Input: part model. Units: mm. Frame: model coordinates. Face numbers are marked on the shaded views. Coordinates: 2 decimals unless noted, no trailing zeros. Write each loop counter-clockwise with the first axis right and the second up, starting at its lowest first coordinate (ties: lowest second). Pieces come first, ordered by that corner, then holes. Notation, with made-up numbers: (-20.5, 31) - (19.5, 31) arc R20 ccw to (19.5, 46) - close; hole circle Ø6 at (41.5, -3). An arc over 180 degrees is marked (long way). One line per question, with ' | ' between items. Start each with the question number.
1) Draft query along Y for the marked faces 1 and 2. Return one class per face: released by +Y, released by -Y, zero draft, split by the parting line, or undercut.
2) First-contact query: P1, Ø1, axis at x = -9, z = 103, coming from the +Y side; P2, Ø5, axis at y = 99, z = 64, coming from the -X side; P3, Ø2.5, axis at x = -9, z = 40.5, coming from the -Y side. Flat tips, straight axial feed; report the tip coordinate or a pass-through.
3) Section query B-B on y = 100. Return loops of the section in (x, z).
4) Line query: line 1 (Y direction, x = -3.9, z = 127.75); line 2 (Z direction, x = -2, y = 79.5); line 3 (X direction, y = 83.5, z = 32.5). Output: solid intervals per line, ascending.
```python
from build123d import *
from OCP.BRepFilletAPI import BRepFilletAPI_MakeChamfer

# Parameters (mm, degrees)
SKETCH1_W           = 95
SKETCH1_H           = 145
BOSS_EXTRUDE1_DEPTH = 10
SKETCH2_W           = 3.3
SKETCH2_H           = 4.8
BOSS_EXTRUDE2_DEPTH = 95
SKETCH3_W           = 3.3
SKETCH3_H           = 149.8
BOSS_EXTRUDE3_DEPTH = 4.9
BOSS_EXTRUDE4_DEPTH = 10
CUT_EXTRUDE1_REACH  = 181.304
SKETCH5_R           = 1.9
SKETCH6_R           = 3.35
CUT_EXTRUDE2_DEPTH  = 2.5
CUT_EXTRUDE3_REACH  = 181.304
SKETCH7_W           = 0.2
SKETCH7_H           = 145
SKETCH8_W           = 85
SKETCH8_H           = 135
CUT_EXTRUDE4_DEPTH  = 5
CHAMFER1_SIZE       = 2.5
CHAMFER1_SIZE_2     = 5


with BuildPart() as part:
    # Sketch1 → Boss-Extrude1 (new body)
    with BuildSketch(Plane.YZ):
        with Locations((47.5, 72.5)):
            Rectangle(SKETCH1_W, SKETCH1_H)
    extrude(amount=-BOSS_EXTRUDE1_DEPTH)

    # Sketch2 → Boss-Extrude2 (add)
    with BuildSketch(Plane.XZ):
        with Locations((-5, -2.4)):
            Rectangle(SKETCH2_W, SKETCH2_H)
    extrude(amount=-BOSS_EXTRUDE2_DEPTH)

    # Sketch3 → Boss-Extrude3 (add)
    with BuildSketch(Plane.XZ):
        with Locations((-5, 70.1)):
            Rectangle(SKETCH3_W, SKETCH3_H)
    extrude(amount=BOSS_EXTRUDE3_DEPTH)

    # Sketch4 → Boss-Extrude4 (add)
    with BuildSketch(Plane(origin=(0, 95, 0), x_dir=(-1, 0, 0), z_dir=(0, 1, 0))):
        Polygon((6.65, 145), (0, 145), (0, 0), (3.35, 0), (6.65, 0), align=None)
    extrude(amount=BOSS_EXTRUDE4_DEPTH)

    # Sketch5 → Cut-Extrude1 (cut, up to next)
    with BuildSketch(Plane.YZ, mode=Mode.PRIVATE) as cut_extrude1_sk1:
        with Locations(Location((100, 127.75, 0), (0, 0, 270))):
            Circle(SKETCH5_R)
    cut_extrude1_tool1 = extrude(cut_extrude1_sk1.sketch, amount=-CUT_EXTRUDE1_REACH, mode=Mode.PRIVATE) & part.part
    add(cut_extrude1_tool1.solids().sort_by_distance((0, 100, 127.75))[0], mode=Mode.SUBTRACT)

    # Sketch6 → Cut-Extrude2 (cut)
    with BuildSketch(Plane.YZ):
        with Locations(Location((100, 127.75, 0), (0, 0, 270))):
            Circle(SKETCH6_R)
    extrude(amount=-CUT_EXTRUDE2_DEPTH, mode=Mode.SUBTRACT)

    # Sketch7 → Cut-Extrude3 (cut, up to next)
    with BuildSketch(Plane.YZ, mode=Mode.PRIVATE) as cut_extrude3_sk1:
        with Locations((104.9, 72.5)):
            Rectangle(SKETCH7_W, SKETCH7_H)
    cut_extrude3_tool1 = extrude(cut_extrude3_sk1.sketch, amount=-CUT_EXTRUDE3_REACH, mode=Mode.PRIVATE) & part.part
    add(cut_extrude3_tool1.solids().sort_by_distance((0, 104.9, 72.5))[0], mode=Mode.SUBTRACT)

    # Sketch8 → Cut-Extrude4 (cut)
    with BuildSketch(Plane(origin=(-10, 0, 0), x_dir=(0, -1, 0), z_dir=(-1, 0, 0))):
        with Locations((-47.5, 72.5)):
            Rectangle(SKETCH8_W, SKETCH8_H)
    extrude(amount=-CUT_EXTRUDE4_DEPTH, mode=Mode.SUBTRACT)

    # Chamfer1
    chamfer1_edges_1 = [part.edges().sort_by_distance(p)[0] for p in [
        (-10, 5, 72.5),
    ]]
    chamfer1_side_1 = [part.faces().sort_by_distance(p)[0] for p in [
        (-10, 4.95, 72.5),
    ]]
    chamfer1_edges_2 = [part.edges().sort_by_distance(p)[0] for p in [
        (-10, 47.5, 5),
    ]]
    chamfer1_side_2 = [part.faces().sort_by_distance(p)[0] for p in [
        (-10, 47.5, 4.95),
    ]]
    chamfer1_edges_3 = [part.edges().sort_by_distance(p)[0] for p in [
        (-10, 90, 72.5),
    ]]
    chamfer1_side_3 = [part.faces().sort_by_distance(p)[0] for p in [
        (-10, 90.05, 72.5),
    ]]
    chamfer1_edges_4 = [part.edges().sort_by_distance(p)[0] for p in [
        (-10, 47.5, 140),
    ]]
    chamfer1_side_4 = [part.faces().sort_by_distance(p)[0] for p in [
        (-10, 47.5, 140.05),
    ]]
    chamfer1 = BRepFilletAPI_MakeChamfer(part.part.solid().wrapped)
    for e in chamfer1_edges_1:
        chamfer1.Add(CHAMFER1_SIZE - 0.0001, CHAMFER1_SIZE_2 - 0.0001, e.wrapped, chamfer1_side_1[0].wrapped)
    for e in chamfer1_edges_2:
        chamfer1.Add(CHAMFER1_SIZE - 0.0001, CHAMFER1_SIZE_2 - 0.0001, e.wrapped, chamfer1_side_2[0].wrapped)
    for e in chamfer1_edges_3:
        chamfer1.Add(CHAMFER1_SIZE - 0.0001, CHAMFER1_SIZE_2 - 0.0001, e.wrapped, chamfer1_side_3[0].wrapped)
    for e in chamfer1_edges_4:
        chamfer1.Add(CHAMFER1_SIZE - 0.0001, CHAMFER1_SIZE_2 - 0.0001, e.wrapped, chamfer1_side_4[0].wrapped)
    add(Compound.cast(chamfer1.Shape()), mode=Mode.REPLACE)  # a hair under: the kernel refuses the full size


solid = part.part
```
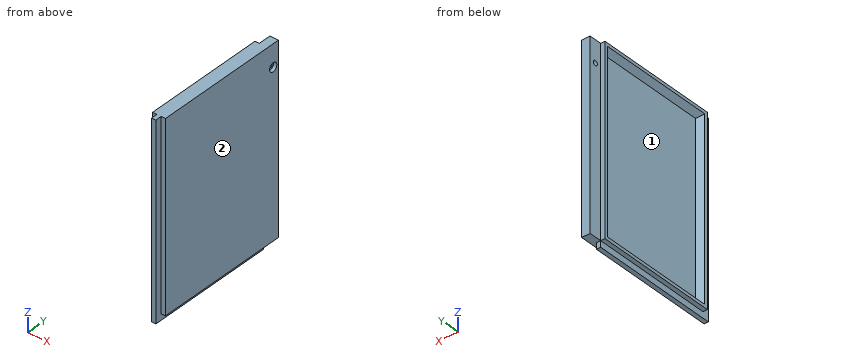
Answer key:
1) face 1: undercut | face 2: zero draft
2) P1: y = 95 | P2: x = -6.65 | P3: y = 0
3) outline: (-6.65, 0) - (0, 0) - (0, 124.4) - (-2.5, 124.4) - (-2.5, 125.85) - (-6.65, 125.85) - close; (-6.65, 129.65) - (-2.5, 129.65) - (-2.5, 131.1) - (0, 131.1) - (0, 145) - (-6.65, 145) - close
4) line 1: -4.9 to 98.1, 101.9 to 104.8 | line 2: 0 to 145 | line 3: -5 to 0
